```python
from build123d import *

# Parameters (mm, degrees)
SKETCH1_W           = 38.1
SKETCH1_H           = 6.35
BOSS_EXTRUDE1_DEPTH = 30.48
SKETCH1_3_W         = 38.1
SKETCH1_3_H         = 38.1
SKETCH1_3_R         = 14.2875
BOSS_EXTRUDE2_DEPTH = 6.35
SKETCH3_W           = 6.35
SKETCH3_H           = 38.1
BOSS_EXTRUDE3_DEPTH = 6.35
BOSS_EXTRUDE4_DEPTH = 2.54
BOSS_EXTRUDE5_DEPTH = 2.54
SKETCH6_R           = 2.413
SKETCH6_R_2         = 2.5796875
CUT_EXTRUDE1_DEPTH  = 7.35


with BuildPart() as part:
    # Sketch1 → Boss-Extrude1 (new body)
    with BuildSketch(Plane(origin=(0, 0, 0), x_dir=(0, 0, -1), z_dir=(1, 0, 0))):
        with Locations((0, -22.225)):
            Rectangle(SKETCH1_W, SKETCH1_H)
    extrude(amount=BOSS_EXTRUDE1_DEPTH)



with BuildPart() as body_2:
    # Sketch1<3> → Boss-Extrude2 (new body)
    with BuildSketch(Plane(origin=(0, 0, 0), x_dir=(0, 0, -1), z_dir=(1, 0, 0))):
        Rectangle(SKETCH1_3_W, SKETCH1_3_H)
        Circle(SKETCH1_3_R, mode=Mode.SUBTRACT)
    extrude(amount=-BOSS_EXTRUDE2_DEPTH)


with BuildPart() as part_1:
    add(part.part)

    add(body_2.part)  # Boss-Extrude3 merges body 2
    # Sketch3 → Boss-Extrude3 (add)
    with BuildSketch(Plane.XZ.offset(19.05)):
        with Locations((-3.175, 0)):
            Rectangle(SKETCH3_W, SKETCH3_H)
    extrude(amount=BOSS_EXTRUDE3_DEPTH)

    # Sketch4 → Boss-Extrude4 (add)
    with BuildSketch(Plane.XY.offset(19.05)):
        Polygon((0, 19.05), (30.48, -19.05), (0, -19.05), align=None)
    extrude(amount=-BOSS_EXTRUDE4_DEPTH)

    # Sketch5 → Boss-Extrude5 (add)
    with BuildSketch(Plane(origin=(0, 0, -19.05), x_dir=(-1, 0, 0), z_dir=(0, 0, -1))):
        Polygon((0, 19.05), (-30.48, -19.05), (0, -19.05), align=None)
    extrude(amount=-BOSS_EXTRUDE5_DEPTH)

    # Sketch6 → Cut-Extrude1 (cut, through all)
    with BuildSketch(Plane(origin=(0, -19.05, 0), x_dir=(1, 0, 0), z_dir=(0, 1, 0))):
        with Locations((7.62, -8.255)):
            Circle(SKETCH6_R)
        with Locations((22.098, -8.255)):
            Circle(SKETCH6_R_2)
        with Locations((22.098, 8.128)):
            Circle(SKETCH6_R)
        with Locations((7.62, 8.128)):
            Circle(SKETCH6_R)
    extrude(amount=-CUT_EXTRUDE1_DEPTH, mode=Mode.SUBTRACT)


solid = part_1.part
```
CAD build for the part. Positions are in the model's coordinates, mm. A direction names the side the tool comes from. Give positions to 0.01 mm unless a question says otherwise; leave off trailing zeros. Order: outer loops, then holes, each group sorted by start corner. A loop starts at its lowest first (then second) coordinate and runs counter-clockwise, first axis right, second up.
(1) Saw through at A-A, the plane z = 0. Give the cut face in (x, y), then the cut area to 3 significant figures.
(2) Saw through at C-C, the plane x = 16. Give the cut face in (y, z), then the cut area to 3 significant figures.
(3) Flat gauge pins, fed straight in: pin 1 (5 mm diameter, centred on x = 5, y = 14.5, fed in from +Z); pin 2 (16.5 mm diameter, centred on y = 4.5, z = -7.5, fed in from +X); pin 3 (1.5 mm diameter, centred on x = 15.5, z = 2, fed in from +Y). Where does each tip first touch, or does it go through?
(4) Tool access for faces 4 (the flat face through (-6.35, -13, -9)), 5 (the flat face through (15, -19.05, 0)): list every direction of +Z, -Z, +X, -X, +Y, -Y with a clear straight run to the whole face (end or side of a thin tool).
(5) Saw through at D-D, the plane x = 7.62. Give the cut face in (y, z) (3 decimals), then the cut area to 3 significant figures.
(6) Mould opens along Z. For faces 1 (the cylindrical face through (5.21, -22.18, 8.15)), 2 (the flat face through (12, -25.4, 0)), 3 (the flat face through (8, -8, 19.05)) say: released by +Z, released by -Z, zero draft, split by the parting line, or undercut.
(7) Drill centre lines: L1, parallel to Z at x = 7.62, y = -22 (3 decimals); L2, parallel to Z at x = 17, y = -18.5; L3, parallel to Y at x = 6, z = 12.5. Where is each one in solid material? Low to high.
(8) Saw through at B-B, the plane y = -12.5. Give the cut face in (x, z).
Results found:
1. outline: (-6.35, -25.4) - (30.48, -25.4) - (30.48, -19.05) - (0, -19.05) - (0, -14.29) - (-6.35, -14.29) - close; (-6.35, 14.29) - (0, 14.29) - (0, 19.05) - (-6.35, 19.05) - close
1. area: 294 mm2
2. outline: (-25.4, -19.05) - (-0.95, -19.05) - (-0.95, -16.51) - (-19.05, -16.51) - (-19.05, 16.51) - (-0.95, 16.51) - (-0.95, 19.05) - (-25.4, 19.05) - close
2. area: 334 mm2
3. pin 1: stops at z = 19.05
3. pin 2: stops at x = 0
3. pin 3: stops at y = -19.05
4. face 4: +Z, -Z, -X, +Y, -Y
4. face 5: +X, +Y
5. outline: (-25.4, -19.05) - (9.525, -19.05) - (9.525, -16.51) - (-19.05, -16.51) - (-19.05, -10.541) - (-25.4, -10.541) - close; (-25.4, -5.715) - (-19.05, -5.715) - (-19.05, 5.842) - (-25.4, 5.842) - close; (-25.4, 10.668) - (-19.05, 10.668) - (-19.05, 16.51) - (9.525, 16.51) - (9.525, 19.05) - (-25.4, 19.05) - close
5. area: 326 mm2
6. face 1: undercut
6. face 2: zero draft
6. face 3: released by +Z
7. L1: z = -19.05 to -10.541, -5.715 to 5.842, 10.668 to 19.05
7. L2: z = -19.05 to -16.51, 16.51 to 19.05
7. L3: y = -25.4 to -19.05
8. outline: (-6.35, -19.05) - (25.24, -19.05) - (25.24, -16.51) - (0, -16.51) - (0, -6.92) - (-6.35, -6.92) - close; (-6.35, 6.92) - (0, 6.92) - (0, 16.51) - (25.24, 16.51) - (25.24, 19.05) - (-6.35, 19.05) - close
